Source: CAD feature listing. Evaluate the final solid. Frame: model axes, mm. A direction names the side the tool comes from. Give positions to 0.01 mm unless a question says otherwise; leave off trailing zeros. Use CSV: the item, a comma, the result in double quotes.
```python
from build123d import *

# Parameters (mm, degrees)
SKETCH11_R              = 3.4
SKETCH11_R_2            = 2.1
NH_H_NH_30X30X2_1_DEPTH = 180


with BuildPart() as part:
    # Sketch11 → Ðnh hình 30X30X2(1) (new body)
    with BuildSketch(Plane.YZ):
        with BuildLine():
            Line((13, -4), (13, -8.25))
            Line((13, -8.25), (9.664213562, -8.25))
            Line((9.664213562, -8.25), (6, -4.585786438))
            Line((6, -4.585786438), (6, -0.519615242))
            Line((6, -0.519615242), (5.7, 0))
            Line((5.7, 0), (6, 0.519615242))
            Line((6, 0.519615242), (6, 4.585786438))
            Line((6, 4.585786438), (9.664213562, 8.25))
            Line((9.664213562, 8.25), (13, 8.25))
            Line((13, 8.25), (13, 4))
            Line((13, 4), (15, 4))
            Line((15, 4), (15, 13))
            ThreePointArc((15, 13), (14.414213562, 14.414213562), (13, 15))
            Line((13, 15), (4, 15))
            Line((4, 15), (4, 13))
            Line((4, 13), (8.25, 13))
            Line((8.25, 13), (8.25, 9.664213562))
            Line((8.25, 9.664213562), (4.585786438, 6))
            Line((4.585786438, 6), (0.519615242, 6))
            Line((0.519615242, 6), (0, 5.7))
            Line((0, 5.7), (-0.519615242, 6))
            Line((-0.519615242, 6), (-4.585786438, 6))
            Line((-4.585786438, 6), (-8.25, 9.664213562))
            Line((-8.25, 9.664213562), (-8.25, 13))
            Line((-8.25, 13), (-4, 13))
            Line((-4, 13), (-4, 15))
            Line((-4, 15), (-13, 15))
            ThreePointArc((-13, 15), (-14.414213562, 14.414213562), (-15, 13))
            Line((-15, 13), (-15, 4))
            Line((-15, 4), (-13, 4))
            Line((-13, 4), (-13, 8.25))
            Line((-13, 8.25), (-9.664213562, 8.25))
            Line((-9.664213562, 8.25), (-6, 4.585786438))
            Line((-6, 4.585786438), (-6, 0.519615242))
            Line((-6, 0.519615242), (-5.7, 0))
            Line((-5.7, 0), (-6, -0.519615242))
            Line((-6, -0.519615242), (-6, -4.585786438))
            Line((-6, -4.585786438), (-9.664213562, -8.25))
            Line((-9.664213562, -8.25), (-13, -8.25))
            Line((-13, -8.25), (-13, -4))
            Line((-13, -4), (-15, -4))
            Line((-15, -4), (-15, -13))
            ThreePointArc((-15, -13), (-14.414213562, -14.414213562), (-13, -15))
            Line((-13, -15), (-4, -15))
            Line((-4, -15), (-4, -13))
            Line((-4, -13), (-8.25, -13))
            Line((-8.25, -13), (-8.25, -9.664213562))
            Line((-8.25, -9.664213562), (-4.585786438, -6))
            Line((-4.585786438, -6), (-0.519615242, -6))
            Line((-0.519615242, -6), (0, -5.7))
            Line((0, -5.7), (0.519615242, -6))
            Line((0.519615242, -6), (4.585786438, -6))
            Line((4.585786438, -6), (8.25, -9.664213562))
            Line((8.25, -9.664213562), (8.25, -13))
            Line((8.25, -13), (4, -13))
            Line((4, -13), (4, -15))
            Line((4, -15), (13, -15))
            ThreePointArc((13, -15), (14.414213562, -14.414213562), (15, -13))
            Line((15, -13), (15, -4))
            Line((15, -4), (13, -4))
        make_face()
        Circle(SKETCH11_R, mode=Mode.SUBTRACT)
        with Locations((11.6, -11.6)):
            Circle(SKETCH11_R_2, mode=Mode.SUBTRACT)
        with Locations((11.6, 11.6)):
            Circle(SKETCH11_R_2, mode=Mode.SUBTRACT)
        with Locations((-11.6, 11.6)):
            Circle(SKETCH11_R_2, mode=Mode.SUBTRACT)
        with Locations((-11.6, -11.6)):
            Circle(SKETCH11_R_2, mode=Mode.SUBTRACT)
    extrude(amount=NH_H_NH_30X30X2_1_DEPTH)


solid = part.part
```
Item 1: First-contact query: pin 1 (1.2 mm diameter, centred on x = 61.5, z = -2, fed in from -Y); pin 2 (0.6 mm diameter, centred on x = 85.5, z = 14, fed in from -Y); pin 3 (2 mm diameter, centred on x = 96, z = -1, fed in from +Y). Flat tips, straight axial feed; report the tip coordinate or a pass-through.
Filled in:
pin 1,"stops at y = -6"
pin 2,"stops at y = -14.87"
pin 3,"stops at y = 6"
Item 2: Mould query, pull axis Z, two halves, no side actions, for faces 1 (the flat face through (89, 15, -9)), 2 (the flat face through (88.74, 7.858, -6.444)), 3 (the flat face through (89, 9, 15)). Classes: released by +Z, released by -Z, zero draft, split by the parting line, or undercut.
Filled in:
face 1,"zero draft"
face 2,"undercut"
face 3,"released by +Z"
Item 3: Material intervals for line 1 (Z direction, x = 134, y = 11.6); line 2 (Y direction, x = 103.5, z = -4.5); line 3 (Y direction, x = 9.5, z = 11.25), sorted ascending. Write a range as from..to.
Filled in:
line 1,"z = -15..-13.7, -9.5..-8.25, 8.25..9.5, 13.7..15"
line 2,"y = -15..-13, -6..6, 13..15"
line 3,"y = -15..-13.67, -9.53..-8.25, 8.25..9.53, 13.67..15"
Item 4: Set-up query: faces 4 (the flat face through (89, -15, 9)), 5 (the flat face through (89, -8.25, -11)). Return all of +Z, -Z, +X, -X, +Y, -Y with unobstructed straight access to the full face (end or side cutting, diameter ignored); none if empty.
Filled in:
face 4,"+Z, -Z, +X, -X, -Y"
face 5,"+X, -X"
Item 5: Section A-A on x = 79. Count the separate pieces of the cut face and the enclosed holes in it, then the cut area to 3 significant figures.
Filled in:
separate pieces,"1"
enclosed holes,"5"
area,"332 mm2"
